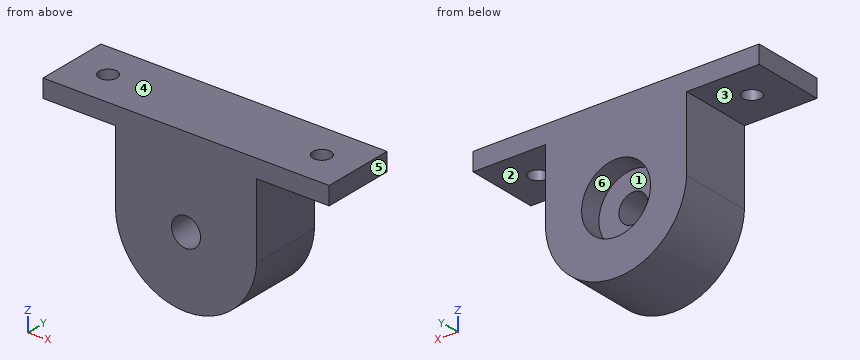
from build123d import *

# Parameters (mm, degrees)
BODY_START           = -20
BODY_OUTLINE_R       = 9.525
BODY_DEPTH           = 20
SKETCH2_R            = 2.5
MOUNTING_HOLES_DEPTH = 5
SKETCH3_R            = 9.525
SKETCH3_R_2          = 4
HOLEINSERT_DEPTH     = 14


# Read off the part's stored shape, not the designer's step: Body
with BuildPart() as part:
    # Body outline → Body (new body)
    with BuildSketch(Plane(origin=(0, 0, 0), x_dir=(1, 0, 0), z_dir=(0, 1, 0)).offset(BODY_START)):
        with BuildLine():
            Line((16.5, 2.5), (16.5, 23.012737313))
            ThreePointArc((16.5, 23.012737313), (-3, 41.55), (-22.5, 23.012737313))
            Line((-22.5, 23.012737313), (-22.5, 2.5))
            Line((-22.5, 2.5), (-42.5, 2.5))
            Line((-42.5, 2.5), (-42.5, -2.5))
            Line((-42.5, -2.5), (36.5, -2.5))
            Line((36.5, -2.5), (36.5, 2.5))
            Line((36.5, 2.5), (16.5, 2.5))
        make_face()
        with Locations((-3, 22.025)):
            Circle(BODY_OUTLINE_R, mode=Mode.SUBTRACT)
    extrude(amount=BODY_DEPTH)

    # Sketch2 → Mounting Holes (cut)
    with BuildSketch(Plane(origin=(0, 0, -2.5), x_dir=(-1, 0, 0), z_dir=(0, 0, -1))):
        with Locations((-26.5, -10)):
            Circle(SKETCH2_R)
        with Locations((32.5, -10)):
            Circle(SKETCH2_R)
    extrude(amount=-MOUNTING_HOLES_DEPTH, mode=Mode.SUBTRACT)

    # Sketch3 → HoleInsert (add)
    with BuildSketch(Plane.XZ.offset(20)):
        with Locations(Location((-3, -22.025, 0), (0, 0, 90))):
            Circle(SKETCH3_R)
        with Locations(Location((-3, -22.025, 0), (0, 0, 270))):
            Circle(SKETCH3_R_2, mode=Mode.SUBTRACT)
    extrude(amount=-HOLEINSERT_DEPTH)


solid = part.part
Geometry: final body of the model. Coordinates: model frame, mm. Face numbers are marked on the shaded views. A direction names the side the tool comes from. Give positions to 0.01 mm unless a question says otherwise; leave off trailing zeros. Order: outer loops, then holes, each group sorted by start corner. A loop starts at its lowest first (then second) coordinate and runs counter-clockwise, first axis right, second up. Notation, with made-up numbers: (31, -37.75) -> (48, -37.75) arc R31 cw to (48, 1.25) -> close; hole circle Ø6 at (-35.75, 63.5). An arc over 180 degrees is marked (long way). Write each question's results on one line, items separated by ' | '.
1) Cut plane D-D (z = -1). Output: boundary loops of the cut face in (x, y), and give its area (3 significant figures).
Geometry says:
outline: (-42.5, -20) -> (36.5, -20) -> (36.5, 0) -> (-42.5, 0) -> close; hole circle Ø5 at (-32.5, -10); hole circle Ø5 at (26.5, -10) | area: 1,540 mm²
2) Cut plane A-A (y = -10). Output: boundary loops of the cut face in (x, z) (3 decimals), and give its area (4 significant figures).
Geometry says:
outline: (-42.5, -2.5) -> (-35, -2.5) -> (-35, 2.5) -> (-42.5, 2.5) -> close; (-30, -2.5) -> (-22.5, -2.5) -> (-22.5, -23.013) arc R19.525 ccw to (16.5, -23.013) -> (16.5, -2.5) -> (24, -2.5) -> (24, 2.5) -> (-30, 2.5) -> close; (29, -2.5) -> (36.5, -2.5) -> (36.5, 2.5) -> (29, 2.5) -> close; hole circle Ø8 at (-3, -22.025) | area: 1,655 mm²
3) Draft query along Z for the marked faces 4, 5 and 6. Return one class per face: released by +Z, released by -Z, zero draft, split by the parting line, or undercut.
Geometry says:
face 4: released by +Z | face 5: zero draft | face 6: undercut
4) Cut plane C-C (y = -17.25). Output: boundary loops of the cut face in (x, z) (3 decimals).
Geometry says:
outline: (-42.5, -2.5) -> (-22.5, -2.5) -> (-22.5, -23.013) arc R19.525 ccw to (16.5, -23.013) -> (16.5, -2.5) -> (36.5, -2.5) -> (36.5, 2.5) -> (-42.5, 2.5) -> close; hole circle Ø8 at (-3, -22.025)
5) First-contact query: pin 1 Ø1.5 at (y, z) = (-5, -35) entering from -X; pin 2 Ø10 at (y, z) = (-12, -13.5) entering from -X; pin 3 Ø10 at (x, y) = (29, -14.5) entering from -Z. Flat tips, straight axial feed; report the tip coordinate or a pass-through.
Geometry says:
pin 1: stops at x = -18.22 | pin 2: stops at x = -22.5 | pin 3: stops at z = -2.5
6) Line query: line 1 along X through (y, z) = (-10.75, -14.5); line 2 along Y through (x, z) = (26.5, 1.4); line 3 along Z through (x, y) = (28.5, -3). Output: solid intervals per line, ascending.
Geometry says:
line 1: x = -22.5 to 16.5 | line 2: y = -20 to -12.5, -7.5 to 0 | line 3: z = -2.5 to 2.5
7) Set-up query: the marked faces 1, 2 and 3. Return all of +Z, -Z, +X, -X, +Y, -Y with unobstructed straight access to the full face (end or side cutting, diameter ignored); none if empty.
Geometry says:
face 1: +Y | face 2: -Z, +X, +Y, -Y | face 3: -Z, -X, +Y, -Y
8) Cut plane B-B (x = -3). Output: boundary loops of the cut face in (y, z) (3 decimals).
Geometry says:
outline: (-20, -41.55) -> (0, -41.55) -> (0, -31.55) -> (-6, -31.55) -> (-6, -26.025) -> (-20, -26.025) -> close; (-20, -18.025) -> (-6, -18.025) -> (-6, -12.5) -> (0, -12.5) -> (0, 2.5) -> (-20, 2.5) -> close
